Verification items for the finished model (mm, model axes). A direction names the side the tool comes from. Round coordinates to 2 decimals unless told otherwise and drop trailing zeros. Order: outer loops, then holes, each group sorted by start corner. A loop starts at its lowest first (then second) coordinate and runs counter-clockwise, first axis right, second up. Notation, with made-up numbers: (64.5, 45.25) -> (80.5, 45.25) arc R34 ccw to (80.5, 76.25) -> close; hole circle Ø1 at (-8.5, 12.5). An arc over 180 degrees is marked (long way). Write item = value, one per line. Start each with the question number.
from build123d import *

# Parameters (mm, degrees)
F0_W        = 50.8
F0_H        = 50.8
F1_DEPTH    = 101.6
F0_W_2      = 76.2
F0_H_2      = 76.2
F0_R        = 3.175
F2_DEPTH    = 12.7
F3_R        = 19.05
F4_DEPTH    = 101.601
F5_R        = 3.175
F6_DEPTH    = 25.4
F7_T1_DEPTH = 88.9
F8_R        = 2.54


# Not quite as in the source:
# - a fillet or chamfer that OpenCascade refuses, or shapes differently, is made with other operations: its cross-section is extruded or revolved along the edge and cut away or added


with BuildPart() as f1:
    # F0 (on Top) → F1 (new body)
    with BuildSketch(Plane.XY):
        Rectangle(F0_W, F0_H)
    extrude(amount=F1_DEPTH)

    # F0 (on Top) → F2 (join)
    with BuildSketch(Plane.XY):
        Rectangle(F0_W_2, F0_H_2)
        with Locations((-31.6072627902, -31.269069761)):
            Circle(F0_R, mode=Mode.SUBTRACT)
        with Locations((31.3326152668, -31.2626581123)):
            Circle(F0_R, mode=Mode.SUBTRACT)
        Rectangle(F0_W, F0_H, mode=Mode.SUBTRACT)
        with Locations((-31.2740796408, 31.5370819021)):
            Circle(F0_R, mode=Mode.SUBTRACT)
        with Locations((31.2819033467, 31.1061042501)):
            Circle(F0_R, mode=Mode.SUBTRACT)
    extrude(amount=F2_DEPTH)

    # F3 (on face) → F4 (cut, through all)
    with BuildSketch(Plane.XY.offset(101.6)):
        Circle(F3_R)
    extrude(amount=-F4_DEPTH, mode=Mode.SUBTRACT)

    # F5 (on face) → F6 (cut)
    with BuildSketch(Plane.YZ.offset(25.4)):
        with Locations((0, 37.7008840442)):
            Circle(F5_R)
    extrude(amount=-F6_DEPTH, mode=Mode.SUBTRACT)

    # F7: fillet of radius 25.4 on 4 edges, made by hand

    # F7_s2 → F7_t1 (cut)
    with BuildSketch(Plane.XY.offset(12.7)):
        with BuildLine():
            ThreePointArc((0, -25.4), (17.9605122421, -17.9605122421), (25.4, 0))
            Line((25.4, 0), (25.908, 0))
            Line((25.908, 0), (25.908, -25.908))
            Line((25.908, -25.908), (0, -25.908))
            Line((0, -25.908), (0, -25.4))
        make_face()
        with BuildLine():
            ThreePointArc((25.4, 0), (17.9605122421, 17.9605122421), (0, 25.4))
            Line((0, 25.4), (0, 25.908))
            Line((0, 25.908), (25.908, 25.908))
            Line((25.908, 25.908), (25.908, 0))
            Line((25.908, 0), (25.4, 0))
        make_face()
        with BuildLine():
            ThreePointArc((0, -25.4), (-17.9605122421, -17.9605122421), (-25.4, 0))
            Line((-25.4, 0), (-25.908, 0))
            Line((-25.908, 0), (-25.908, -25.908))
            Line((-25.908, -25.908), (0, -25.908))
            Line((0, -25.908), (0, -25.4))
        make_face()
        with BuildLine():
            ThreePointArc((-25.4, 0), (-17.9605122421, 17.9605122421), (0, 25.4))
            Line((0, 25.4), (0, 25.908))
            Line((0, 25.908), (-25.908, 25.908))
            Line((-25.908, 25.908), (-25.908, 0))
            Line((-25.908, 0), (-25.4, 0))
        make_face()
    extrude(amount=F7_T1_DEPTH, mode=Mode.SUBTRACT)

    # F8
    f8_edges = [f1.edges().sort_by_distance(p)[0] for p in [
        (0, -38.1, 12.7),
        (38.1, 0, 12.7),
        (-38.1, 0, 12.7),
        (0, 38.1, 12.7),
    ]]
    fillet(f8_edges, radius=F8_R)


solid = f1.part
(1) Cross-section at C-C (z = 76). Enter the section's corners in (x, y), and give its area (3 significant figures).
(2) Cross-section at B-B (x = 33). Enter the section's corners in (y, z), and give its area (3 significant figures).
(3) Cross-section at A-A (y = 9). Enter the section's corners in (x, z), and give its area (3 significant figures).
(4) Cross-section at D-D (x = 22). Enter the section's corners in (y, z) (3 decimals).
(5) Scan lines: line 1 along Y through (x, z) = (0, 47); line 2 along Z through (x, y) = (28, 17); line 3 along X through (y, z) = (5.5, 57). Record each from-to range of solid material in increasing order. Write a range as from..to.
(6) Set-up check for faces 1 (the cylindrical face through (22.138, 1.707, 40.378)), 2 (the flat face through (-38.1, -1, 5)), 3 (the flat face through (-8.4, 24.2, 12.7)): record each of +Z, -Z, +X, -X, +Y, -Y from which the full face is reachable in a straight line by a thin tool's end or side.
(7) Depth check by flat-ended pin: pin 1 (1.5 mm diameter, centred on x = -11, y = -14, fed in from +Z); pin 2 (10 mm diameter, centred on x = 1, z = 65.5, fed in from -Y); pin 3 (4 mm diameter, centred on x = 5, z = 69, fed in from +Y); pin 4 (5 mm diameter, centred on y = -6, z = 72.5, fed in from -X). Enter the tip coordinate at first touch or a pass-through.
(8) Draft check along X on faces 4 (the flat face through (-9, 17, 0)), 5 (the cylindrical face through (-37.376, 0.533, 11.936)), 6 (the cylindrical face through (-15.12, -11.59, 51.51)). Enter one of: +X half, -X half, draft (parallel to the pull), parting line (faces both ways), or undercut.
Outcome:
q1.outline = circle Ø50.8 at (0, 0); hole circle Ø38.1 at (0, 0)
q1.area = 887 mm^2
q2.outline = (-38.1, 0) -> (-33.96, 0) -> (-33.96, 12.7) -> (-35.56, 12.7) arc R2.54 ccw to (-38.1, 10.16) -> close; (-28.56, 0) -> (28.44, 0) -> (28.44, 12.7) -> (-28.56, 12.7) -> close; (33.78, 0) -> (38.1, 0) -> (38.1, 10.16) arc R2.54 ccw to (35.56, 12.7) -> (33.78, 12.7) -> close
q2.area = 829 mm^2
q3.outline = (-38.1, 0) -> (-16.79, 0) -> (-16.79, 101.6) -> (-23.75, 101.6) -> (-23.75, 12.7) -> (-35.56, 12.7) arc R2.54 ccw to (-38.1, 10.16) -> close; (16.79, 0) -> (38.1, 0) -> (38.1, 10.16) arc R2.54 ccw to (35.56, 12.7) -> (23.75, 12.7) -> (23.75, 101.6) -> (16.79, 101.6) -> close
q3.area = 1,780 mm^2
q4.outline = (-38.1, 0) -> (38.1, 0) -> (38.1, 10.16) arc R2.54 ccw to (35.56, 12.7) -> (12.695, 12.7) -> (12.695, 101.6) -> (-12.695, 101.6) -> (-12.695, 12.7) -> (-35.56, 12.7) arc R2.54 ccw to (-38.1, 10.16) -> close; hole circle Ø6.35 at (0, 37.701)
q5.line_1 = -25.4..-19.05, 19.05..25.4
q5.line_2 = 0..12.7
q5.line_3 = -24.8..-18.24, 18.24..24.8
q6.face_1 = +X
q6.face_2 = +Z, -Z, -X, +Y, -Y
q6.face_3 = +Z
q7.pin_1 = through
q7.pin_2 = -25.4
q7.pin_3 = 25.22
q7.pin_4 = -25.16
q8.face_4 = draft
q8.face_5 = -X half
q8.face_6 = undercut
